The listing builds one solid part. Answer for the finished solid, in the listing's coordinates (mm). Face numbers are marked on the shaded views. Coordinates: 2 decimals unless noted, no trailing zeros. Write each loop counter-clockwise with the first axis right and the second up, starting at its lowest first coordinate (ties: lowest second). Pieces come first, ordered by that corner, then holes.
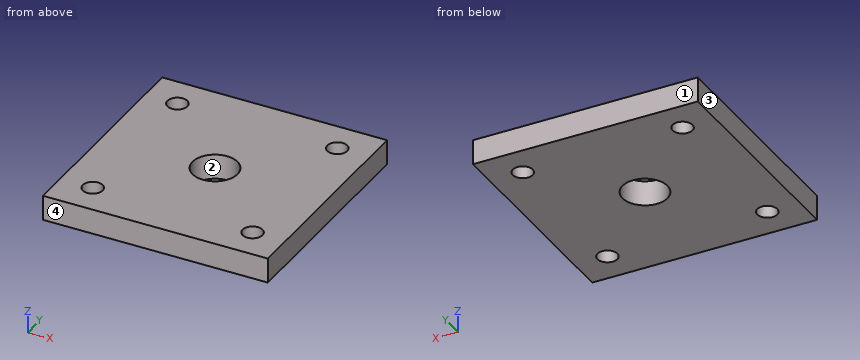
from build123d import *

# Parameters (mm, degrees)
SKETCH1_W           = 45
SKETCH1_H           = 45
SKETCH1_R           = 4.5
BOSS_EXTRUDE1_DEPTH = 5
CUT_EXTRUDE1_DEPTH  = 532.736885204


with BuildPart() as part:
    # Sketch1 → Boss-Extrude1 (new body)
    with BuildSketch(Plane.XY):
        Rectangle(SKETCH1_W, SKETCH1_H)
        Circle(SKETCH1_R, mode=Mode.SUBTRACT)
    extrude(amount=BOSS_EXTRUDE1_DEPTH)

    # Sketch2 → Cut-Extrude1 (cut, through all)
    with BuildSketch(Plane(origin=(-496.037536649, -95.134766003, 0), x_dir=(-1, 0, 0), z_dir=(0, 0, -1))):
        with BuildLine():
            ThreePointArc((-510.037536649, 79.134766003), (-512.037536649, 81.134766003), (-514.037536649, 79.134766003))
            ThreePointArc((-514.037536649, 79.134766003), (-512.037536649, 77.134766003), (-510.037536649, 79.134766003))
        make_face()
        with BuildLine():
            ThreePointArc((-478.037536649, 79.134766003), (-480.037536649, 81.134766003), (-482.037536649, 79.134766003))
            ThreePointArc((-482.037536649, 79.134766003), (-480.037536649, 77.134766003), (-478.037536649, 79.134766003))
        make_face()
        with BuildLine():
            ThreePointArc((-478.037536649, 111.134766003), (-480.037536649, 113.134766003), (-482.037536649, 111.134766003))
            ThreePointArc((-482.037536649, 111.134766003), (-480.037536649, 109.134766003), (-478.037536649, 111.134766003))
        make_face()
        with BuildLine():
            ThreePointArc((-510.037536649, 111.134766003), (-512.037536649, 113.134766003), (-514.037536649, 111.134766003))
            ThreePointArc((-514.037536649, 111.134766003), (-512.037536649, 109.134766003), (-510.037536649, 111.134766003))
        make_face()
    extrude(amount=-CUT_EXTRUDE1_DEPTH, mode=Mode.SUBTRACT)


solid = part.part
Q1. The part is cut by section C-C, the plane z = 1.05. Write down the section's boundary in (x, y), then the cut area to 3 significant figures.
Answers below:
outline: (-22.5, -22.5) - (22.5, -22.5) - (22.5, 22.5) - (-22.5, 22.5) - close; hole circle Ø4 at (-16, -16); hole circle Ø4 at (-16, 16); hole circle Ø9 at (0, 0); hole circle Ø4 at (16, -16); hole circle Ø4 at (16, 16)
area: 1,910 mm2
Q2. The part is cut by section A-A, the plane x = -16. Write down the section's boundary in (y, z), then the cut area to 3 significant figures.
Answers below:
outline: (-22.5, 0) - (-18, 0) - (-18, 5) - (-22.5, 5) - close; (-14, 0) - (14, 0) - (14, 5) - (-14, 5) - close; (18, 0) - (22.5, 0) - (22.5, 5) - (18, 5) - close
area: 185 mm2
Q3. The part is cut by section D-D, the plane x = 0. Write down the section's boundary in (y, z).
Answers below:
outline: (-22.5, 0) - (-4.5, 0) - (-4.5, 5) - (-22.5, 5) - close; (4.5, 0) - (22.5, 0) - (22.5, 5) - (4.5, 5) - close
Q4. Determine the mould class of the marked faces 1, 2, 3 and 4 for opening direction Y: released by +Y, released by -Y, zero draft, split by the parting line, or undercut.
Answers below:
face 1: released by +Y
face 2: undercut
face 3: zero draft
face 4: released by -Y
Q5. Find the intervals of material crossed by probe 1 along Y at (x, z) = (16, 2.05); probe 2 along X at (y, z) = (-15, 1), in increasing order.
Answers below:
probe 1: y = -22.5 to -18, -14 to 14, 18 to 22.5
probe 2: x = -22.5 to -17.73, -14.27 to 14.27, 17.73 to 22.5
Q6. Given pin 1 (3 mm diameter, centred on x = 16, y = -16, fed in from -Z), flat-ended and moving along its own axis, determine where the tip first touches the part or whether it passes through.
Answers below:
pin 1: passes through
